from build123d import *

# Parameters (mm, degrees)
SKETCH2_R           = 2.4384
SKETCH2_R_2         = 4.66725
BOSS_EXTRUDE1_DEPTH = 7.9375


with BuildPart() as part:
    # Sketch2 → Boss-Extrude1 (new body)
    with BuildSketch(Plane(origin=(0, 0, 0), x_dir=(1, 0, 0), z_dir=(0, 1, 0))):
        with BuildLine():
            Line((55.590698865, -86.917376556), (57.091379829, -86.917376556))
            Line((57.091379829, -86.917376556), (83.572039589, -60.436716796))
            ThreePointArc((83.572039589, -60.436716796), (92.583392677, -60.167850758), (99.145825273, -53.986325716))
            Line((99.145825273, -53.986325716), (133.917161076, -54.4991448))
            ThreePointArc((133.917161076, -54.4991448), (134.310699941, -48.951866676), (134.040463462, -43.397216403))
            Line((134.040463462, -43.397216403), (99.145825273, -42.882578814))
            ThreePointArc((99.145825273, -42.882578814), (94.154259421, -37.482880814), (87.006822934, -35.754696848))
            Line((87.006822934, -35.754696848), (70.035827706, -5.332650295))
            ThreePointArc((70.035827706, -5.332650295), (65.026183263, -7.747234822), (60.339928944, -10.741525445))
            Line((60.339928944, -10.741525445), (77.310924172, -41.163571998))
            ThreePointArc((77.310924172, -41.163571998), (75.144838741, -46.683971579), (75.721358625, -52.586035832))
            Line((75.721358625, -52.586035832), (49.240698865, -79.066695593))
            Line((49.240698865, -79.066695593), (49.240698865, -80.567376556))
            ThreePointArc((49.240698865, -80.567376556), (51.100570805, -85.057504617), (55.590698865, -86.917376556))
        make_face()
        with Locations(Location((58.765698865, -77.392376556, 0), (0, 0, 270))):
            Circle(SKETCH2_R, mode=Mode.SUBTRACT)
        with Locations(Location((87.723623157, -48.434452265, 0), (0, 0, 270))):
            Circle(SKETCH2_R_2, mode=Mode.SUBTRACT)
        with Locations(Location((127.089342108, -49.015030821, 0), (0, 0, 270))):
            Circle(SKETCH2_R, mode=Mode.SUBTRACT)
        with Locations(Location((68.54355946, -14.052450337, 0), (0, 0, 270))):
            Circle(SKETCH2_R, mode=Mode.SUBTRACT)
    extrude(amount=BOSS_EXTRUDE1_DEPTH)


solid = part.part
Design review of the part built by this model. Coordinates are the model's own, in mm. A direction names the side the tool comes from. Give positions to 0.01 mm unless a question says otherwise; leave off trailing zeros. Loops run counter-clockwise (first coordinate to the right, second up) from the corner with the lowest first, then second, coordinate; pieces in that order, holes last. Notation, with made-up numbers: M 77.25,-30 L 90.25,-30 A27 ccw 90.25,0 Z; hole C 79.5,21.25 d9. An arc over 180 degrees is marked long. One line per question, with ' | ' between items. Start each with the question number.
1. Add section A-A (x = 74). Write out the cut boundary in (y, z).
2. For faces 1 (the face through (57.832, 3.913, 79.645)), 2 (the face through (62.67, 3.91, 65.64)), list the 3-axis set-ups (+Z, -Z, +X, -X, +Y, -Y) from which the entire face can be reached by the end or side of a thin tool; tool diameter is ignored.
3. Insertion check: P1, Ø4, axis at x = 68.5, y = 4, coming from the -Z side. The pin has a flat end and moves straight along its axis. Give the tip position at first contact, or say it passes through.
4. The part is to be moulded in two halves that separate along Z. For faces 3 (the face through (134.31, 3.91, 49.03)), 4 (the face through (68.707, 3.913, 25.74)), 5 (the face through (82, 7.938, 49)), 6 (the face through (70.15, 3.91, 73.86)), say which applies: released by +Z, released by -Z, zero draft, split by the parting line, or undercut.
5. Add section C-C (y = 5). Write out the cut boundary in (x, z), plus the area to 3 significant figures.
6. To check wall thickness, follow L1, parallel to Z at x = 64, y = 1; L2, parallel to Z at x = 88, y = 5; L3, parallel to X at y = 6.25, z = 15. State the ranges of each line that lie inside material, in increasing order.
7. Add section B-B (z = 76.5). Write out the cut boundary in (x, y), plus the area to 3 significant figures.
8. Add section D-D (x = 109.5). Write out the cut boundary in (y, z).
Worked out:
1) outline: M 0,12.44 L 7.94,12.44 L 7.94,35.23 L 0,35.23 Z; M 0,54.31 L 7.94,54.31 L 7.94,70.01 L 0,70.01 Z
2) face 1: +Y, -Y | face 2: -X, +Y, -Y
3) P1: stops at z = 5.33
4) face 3: split by the parting line | face 4: undercut | face 5: zero draft | face 6: released by +Z
5) outline: M 49.24,79.07 L 75.72,52.59 A12.7 ccw 77.31,41.16 L 60.34,10.74 A46.59 ccw 70.04,5.33 L 87.01,35.75 A12.7 ccw 99.15,42.88 L 134.04,43.4 A46.59 ccw 133.92,54.5 L 99.15,53.99 A12.7 ccw 83.57,60.44 L 57.09,86.92 L 55.59,86.92 A6.35 ccw 49.24,80.57 Z; hole C 58.77,77.39 d4.88; hole C 68.54,14.05 d4.88; hole C 87.72,48.43 d9.33; hole C 127.09,49.02 d4.88 | area: 1,570 mm²
6) L1: z = 8.34 to 17.3, 64.31 to 80.01 | L2: z = 35.74 to 43.78, 53.09 to 61.13 | L3: x = 62.72 to 66.3, 70.79 to 75.43
7) outline: M 51.81,0 L 56.5,0 L 56.5,7.94 L 51.81,7.94 Z; M 61.03,0 L 67.51,0 L 67.51,7.94 L 61.03,7.94 Z | area: 88.6 mm²
8) outline: M 0,43.04 L 7.94,43.04 L 7.94,54.14 L 0,54.14 Z
